from build123d import *

# Parameters (mm, degrees)
PAD_DEPTH    = 22
PAD001_DEPTH = 5
FILLET_R     = 4


with BuildPart() as part:
    # Sketch → Pad (new body)
    with BuildSketch(Plane.XY):
        with BuildLine():
            Line((-15.033203, -2.996852), (-15.033203, 2.868629))
            ThreePointArc((-13.935943, 3.965889), (-14.711823, 3.644509), (-15.033203, 2.868629))
            Line((-13.935943, 3.965889), (13.869538, 3.965889))
            ThreePointArc((14.966797, 2.868629), (14.645418, 3.644509), (13.869538, 3.965889))
            Line((14.966797, 2.868629), (14.966797, -2.996852))
            ThreePointArc((13.869538, -4.094111), (14.645418, -3.772731), (14.966797, -2.996852))
            Line((13.869538, -4.094111), (-13.935943, -4.094111))
            ThreePointArc((-15.033203, -2.996852), (-14.711823, -3.772731), (-13.935943, -4.094111))
        make_face()
        with BuildLine():
            Line((-11.363415, -0.882751), (-11.363415, 0.807684))
            ThreePointArc((-11.083632, 1.087466), (-11.281469, 1.00552), (-11.363415, 0.807684))
            Line((-11.083632, 1.087466), (11.126802, 1.087466))
            ThreePointArc((11.406585, 0.807684), (11.324638, 1.00552), (11.126802, 1.087466))
            Line((11.406585, 0.807684), (11.406585, -0.882751))
            ThreePointArc((11.126802, -1.162534), (11.324638, -1.080587), (11.406585, -0.882751))
            Line((11.126802, -1.162534), (-11.083632, -1.162534))
            ThreePointArc((-11.363415, -0.882751), (-11.281469, -1.080587), (-11.083632, -1.162534))
        make_face(mode=Mode.SUBTRACT)
    extrude(amount=PAD_DEPTH)

    # Sketch001 (on Face18 of Pad) → Pad001 (join)
    with BuildSketch(Plane.XY.offset(22)):
        with BuildLine():
            Line((15.12127, -2.809895), (15.12127, 2.736811))
            ThreePointArc((15.12127, 2.736811), (14.753207, 3.625395), (13.864623, 3.993458))
            Line((13.864623, 3.993458), (-13.622083, 3.993458))
            ThreePointArc((-13.622083, 3.993458), (-14.510667, 3.625395), (-14.87873, 2.736811))
            Line((-14.87873, 2.736811), (-14.87873, -2.809895))
            ThreePointArc((-14.87873, -2.809895), (-14.510667, -3.698479), (-13.622083, -4.066542))
            Line((-13.622083, -4.066542), (13.864623, -4.066542))
            ThreePointArc((13.864623, -4.066542), (14.753207, -3.698479), (15.12127, -2.809895))
        make_face()
    extrude(amount=PAD001_DEPTH)

    # Fillet
    fillet_edges = [part.edges().sort_by_distance(p)[0] for p in [
        (15.12127, -0.036542, 27),
        (14.753207, 3.625395, 27),
        (0.12127, 3.993458, 27),
        (-14.510667, 3.625395, 27),
        (-14.87873, -0.036542, 27),
        (-14.510667, -3.698479, 27),
        (0.12127, -4.066542, 27),
        (14.753207, -3.698479, 27),
    ]]
    fillet(fillet_edges, radius=FILLET_R)


solid = part.part
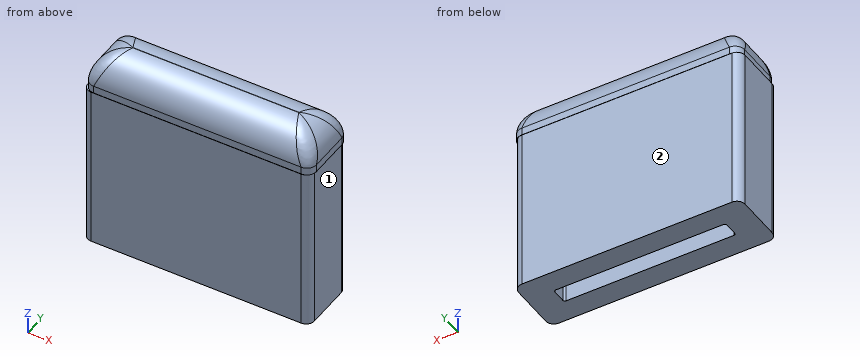
Verification items for the finished model (mm, model axes). Face numbers are marked on the shaded views. A direction names the side the tool comes from. Coordinates: 2 decimals unless noted, no trailing zeros. Loops run counter-clockwise (first coordinate to the right, second up) from the corner with the lowest first, then second, coordinate; pieces in that order, holes last. Notation, with made-up numbers: (70, 68.5) -> (120, 68.5) arc R34 ccw to (120, 101.5) -> close; hole circle Ø11 at (32.5, 80.5). An arc over 180 degrees is marked (long way). Answer as a JSON object with one key per item and string values. Group by question number.
Item 1: Sectioned sample at B-B on z = 18.25. Record the boundary of the cut face in (x, y).
Item 2: Depth check by flat-ended pin: pin 1 (1.5 mm diameter, centred on x = -3, y = 1.5, fed in from +Z); pin 2 (2 mm diameter, centred on x = 7, z = 4.5, fed in from +Y); pin 3 (1.4 mm diameter, centred on y = 0, z = 14.5, fed in from +X). Enter the tip coordinate at first touch or a pass-through.
Item 3: Tool access check on the marked faces 1 and 2. Record the directions out of +Z, -Z, +X, -X, +Y, -Y that give a thin tool (end or side, any length) a straight path to the whole face; none if there is none.
Item 4: Scan lines: probe 1 along X at (y, z) = (0.75, 7.5); probe 2 along Y at (x, z) = (3, 8.5); probe 3 along Y at (x, z) = (-13, 5). Record each from-to range of solid material in increasing order.
Evaluation:
{
 "1": {"outline": "(-15.03, -3) arc R1.1 ccw to (-13.94, -4.09) -> (13.87, -4.09) arc R1.1 ccw to (14.97, -3) -> (14.97, 2.87) arc R1.1 ccw to (13.87, 3.97) -> (-13.94, 3.97) arc R1.1 ccw to (-15.03, 2.87) -> close; hole (-11.36, -0.88) arc R0.28 ccw to (-11.08, -1.16) -> (11.13, -1.16) arc R0.28 ccw to (11.41, -0.88) -> (11.41, 0.81) arc R0.28 ccw to (11.13, 1.09) -> (-11.08, 1.09) arc R0.28 ccw to (-11.36, 0.81) -> close"},
 "2": {"pin 1": "stops at z = 26.93", "pin 2": "stops at y = 3.97", "pin 3": "stops at x = 14.97"},
 "3": {"face 1": "-Z, +X, +Y, -Y", "face 2": "-Z, +X, -X, +Y"},
 "4": {"probe 1": "x = -15.03 to -11.36, 11.41 to 14.97", "probe 2": "y = -4.09 to -1.16, 1.09 to 3.97", "probe 3": "y = -4.09 to 3.97"}
}
